```python
from build123d import *

# Parameters (mm, degrees)
SKETCH2_W           = 50
SKETCH2_H           = 50
BOSS_EXTRUDE1_DEPTH = 3
SKETCH3_R           = 1.6
CUT_EXTRUDE1_DEPTH  = 3
FILLET1_R           = 4
SKETCH4_W           = 50
SKETCH4_H           = 3
BOSS_EXTRUDE2_DEPTH = 3
SKETCH5_W           = 3
SKETCH5_H           = 50
BOSS_EXTRUDE3_DEPTH = 55
SKETCH6_W           = 3
SKETCH6_H           = 50
BOSS_EXTRUDE4_DEPTH = 50
SKETCH7_R           = 1.6
CUT_EXTRUDE2_DEPTH  = 3
FILLET2_R           = 4
FILLET3_R           = 3
FILLET4_R           = 6
BOSS_EXTRUDE5_DEPTH = 12.5
FILLET5_R           = 5
FILLET6_R           = 10


with BuildPart() as part:
    # Sketch2 → Boss-Extrude1 (new body)
    with BuildSketch(Plane(origin=(0, 0, 0), x_dir=(1, 0, 0), z_dir=(0, 1, 0))):
        Rectangle(SKETCH2_W, SKETCH2_H)
    extrude(amount=BOSS_EXTRUDE1_DEPTH)

    # Sketch3 → Cut-Extrude1 (cut)
    with BuildSketch(Plane(origin=(0, 3, 0), x_dir=(1, 0, 0), z_dir=(0, 1, 0))):
        with Locations(Location((-20, 20, 0), (0, 0, 270))):
            Circle(SKETCH3_R)
        with Locations(Location((20, 20, 0), (0, 0, 270))):
            Circle(SKETCH3_R)
        with Locations(Location((-20, -20, 0), (0, 0, 270))):
            Circle(SKETCH3_R)
        with Locations(Location((20, -20, 0), (0, 0, 270))):
            Circle(SKETCH3_R)
    extrude(amount=-CUT_EXTRUDE1_DEPTH, mode=Mode.SUBTRACT)

    # Fillet1
    fillet1_edges = [part.edges().sort_by_distance(p)[0] for p in [
        (25, 1.5, 25),
        (25, 1.5, -25),
    ]]
    fillet(fillet1_edges, radius=FILLET1_R)

    # Sketch4 → Boss-Extrude2 (add)
    with BuildSketch(Plane.ZY.offset(25)):
        with Locations((0, 1.5)):
            Rectangle(SKETCH4_W, SKETCH4_H)
    extrude(amount=BOSS_EXTRUDE2_DEPTH)

    # Sketch5 → Boss-Extrude3 (add)
    with BuildSketch(Plane(origin=(0, 3, 0), x_dir=(1, 0, 0), z_dir=(0, 1, 0))):
        with Locations((-26.5, 0)):
            Rectangle(SKETCH5_W, SKETCH5_H)
    extrude(amount=BOSS_EXTRUDE3_DEPTH)

    # Sketch6 → Boss-Extrude4 (add)
    with BuildSketch(Plane(origin=(0, 58, 0), x_dir=(1, 0, 0), z_dir=(0, 1, 0))):
        with Locations((-26.5, 0)):
            Rectangle(SKETCH6_W, SKETCH6_H)
    extrude(amount=BOSS_EXTRUDE4_DEPTH)

    # Sketch7 → Cut-Extrude2 (cut)
    with BuildSketch(Plane(origin=(-25, 0, 0), x_dir=(0, 0, -1), z_dir=(1, 0, 0))):
        with Locations((-20, 63)):
            Circle(SKETCH7_R)
        with Locations((-20, 103)):
            Circle(SKETCH7_R)
        with Locations((20, 103)):
            Circle(SKETCH7_R)
        with Locations((20, 63)):
            Circle(SKETCH7_R)
    extrude(amount=-CUT_EXTRUDE2_DEPTH, mode=Mode.SUBTRACT)

    # Fillet2
    fillet2_edges = [part.edges().sort_by_distance(p)[0] for p in [
        (-26.5, 108, 25),
        (-26.5, 108, -25),
    ]]
    fillet(fillet2_edges, radius=FILLET2_R)

    # Fillet3
    fillet3_edges = [part.edges().sort_by_distance(p)[0] for p in [
        (-25, 3, 0),
    ]]
    fillet(fillet3_edges, radius=FILLET3_R)

    # Fillet4
    fillet4_edges = [part.edges().sort_by_distance(p)[0] for p in [
        (-28, 0, 0),
    ]]
    fillet(fillet4_edges, radius=FILLET4_R)

    # Sketch8 → Boss-Extrude5 (add, symmetric)
    with BuildSketch(Plane.XY):
        Polygon((-2.068537635, 3), (1.068537635, 3), (-25, 88.266344583), (-25, 78.005433723), align=None)
    extrude(amount=BOSS_EXTRUDE5_DEPTH, both=True)

    # Fillet5
    fillet5_edges = [part.edges().sort_by_distance(p)[0] for p in [
        (-25, 83.135889153, -12.5),
        (-25, 88.266344583, 0),
        (-25, 78.005433723, 0),
        (-25, 83.135889153, 12.5),
    ]]
    fillet(fillet5_edges, radius=FILLET5_R)

    # Fillet6
    fillet6_edges = [part.edges().sort_by_distance(p)[0] for p in [
        (1.068537635, 3, 0),
        (-0.5, 3, -12.5),
        (-2.068537635, 3, 0),
        (-0.5, 3, 12.5),
    ]]
    fillet(fillet6_edges, radius=FILLET6_R)


solid = part.part
```
Here's how the part is built. I have some questions about the finished solid (model axes, mm). A direction names the side the tool comes from. Round coordinates to 2 decimals unless told otherwise and drop trailing zeros. Order: outer loops, then holes, each group sorted by start corner. A loop starts at its lowest first (then second) coordinate and runs counter-clockwise, first axis right, second up. Notation, with made-up numbers: M 21,0 L 31,0 A27 ccw 31,32 Z; hole C -18.75,33 d7. An arc over 180 degrees is marked long. Answer in a Markdown table with one row per item.
Item 1: Imagine slicing it at C-C, the plane x = 16. Write out the boundary of the cut face in (y, z), and give its area (3 significant figures).
A:
| item | result |
|---|---|
| outline | M 0,-25 L 3,-25 L 3,25 L 0,25 Z |
| area | 150 mm2 |
Item 2: For faces 4 (the face through (-3.389, 3.984, -18.174)), 5 (the face through (-24.14, 3.9, -0.35)), 6 (the face through (-12.77, 48.27, 0.22)), 7 (the face through (-18.414, 1.521, 19.792)), 8 (the face through (-3.389, 3.984, 18.174)), which set-ups out of +Z, -Z, +X, -X, +Y, -Y let a thin tool reach every point of the face, with its end or its side?
A:
| item | result |
|---|---|
| face 4 | -Z, +X, +Y |
| face 5 | +Z, -Z |
| face 6 | +Z, -Z, +X, +Y |
| face 7 | +Y, -Y |
| face 8 | +Z, +X, +Y |
Item 3: If I drill on L1, parallel to Z at x = -27.1, y = 103; L2, parallel to X at y = 1, z = -20; L3, parallel to Y at x = 5, z = -22.5, over which ranges is the centre line in solid material (lowest first)? Write a range as from..to.
A:
| item | result |
|---|---|
| L1 | z = -25..-21.6, -18.4..18.4, 21.6..25 |
| L2 | x = -25.32..-21.6, -18.4..18.4, 21.6..25 |
| L3 | y = 0..3 |
Item 4: Imagine slicing it at B-B, the plane y = 63. Write out the boundary of the cut face in (x, z).
A:
| item | result |
|---|---|
| outline | M -28,-25 L -25,-25 L -25,-21.6 L -28,-21.6 Z; M -28,-18.4 L -25,-18.4 L -25,-17.5 A5 cw -20,-12.5 L -17.28,-12.5 L -17.28,12.5 L -20,12.5 A5 cw -25,17.5 L -25,18.4 L -28,18.4 Z; M -28,21.6 L -25,21.6 L -25,25 L -28,25 Z |
Item 5: I'm going to push flat-ended pins straight in: pin 1 (20 mm diameter, centred on x = -14, y = 53, fed in from -Z); pin 2 (3.5 mm diameter, centred on x = 20, z = -20, fed in from -Y); pin 3 (9 mm diameter, centred on x = -7.5, y = 31, fed in from +Z); pin 4 (3.5 mm diameter, centred on x = -20, z = 20, fed in from +Y). Where does each tip first touch, or does it pass through?
A:
| item | result |
|---|---|
| pin 1 | stops at z = -14.5 |
| pin 2 | stops at y = 0 |
| pin 3 | stops at z = 12.5 |
| pin 4 | stops at y = 3 |
Item 6: Imagine slicing it at A-A, the plane z = 6. Write out the boundary of the cut face in (x, y).
A:
| item | result |
|---|---|
| outline | M -28,6 A6 ccw -22,0 L 25,0 L 25,3 L 8.47,3 A10 cw -1.09,10.08 L -24.78,87.55 A5 cw -25,89.01 L -25,108 L -28,108 Z; hole M -25,6 A3 ccw -22,3 L -15.58,3 A10 ccw -6.02,15.92 L -15.22,46.01 A5 ccw -25,44.55 Z |
Item 7: Thinking about a two-plate mould opening in X: for faces 1 (the face through (12, 3, 0)), 2 (the face through (25, 1, 0)), 3 (the face through (-13, 43, -12.5)), which applies, +X half, -X half, draft (parallel to the pull), parting line (faces both ways), or undercut?
A:
| item | result |
|---|---|
| face 1 | undercut |
| face 2 | +X half |
| face 3 | draft |
Item 8: Imagine slicing it at D-D, the plane y = 28.5. Write out the boundary of the cut face in (x, z).
A:
| item | result |
|---|---|
| outline | M -28,-25 L -25,-25 L -25,25 L -28,25 Z; M -9.86,-12.5 L -6.73,-12.5 L -6.73,12.5 L -9.86,12.5 Z |
